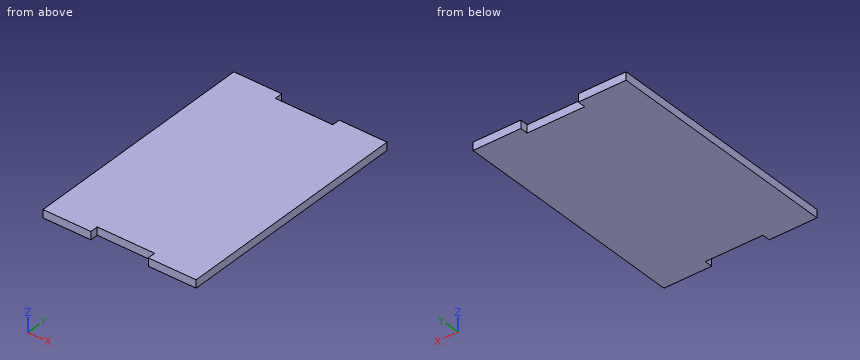
Autodesk Inventor part; units mm, degrees
ref_plane "YZ Plane" through (0, 0, 0) normal (1, 0, 0) x (0, 1, 0)
ref_plane "XZ Plane" through (0, 0, 0) normal (0, 1, 0) x (-1, 0, 0)
ref_plane "XY Plane" through (0, 0, 0) normal (0, 0, 1) x (1, 0, 0)
sketch "Sketch1" plane through (0, 0, 0) normal (0, 0, 1) x (1, 0, 0)
  line L0 (0, 2.8582) -> (0, -2.8582) construction
  line L1 (-5.7775, 0) -> (5.7775, 0) construction
  line L2 (0, 0) -> (96, 0)
  line L3 (96, 0) -> (96, -150)
  line L4 (96, -150) -> (0, -150)
  line L5 (0, -150) -> (0, 0)
  line L6 (0, 0) -> (30, 0)
  line L7 (30, 0) -> (66, 0)
  line L8 (0, -150) -> (30, -150)
  line L9 (30, 0) -> (66, 0)
  line L10 (66, 0) -> (66, -5)
  line L11 (66, -5) -> (30, -5)
  line L12 (30, -5) -> (30, 0)
  line L13 (30, -150) -> (66, -150)
  line L14 (66, -150) -> (66, -145)
  line L15 (66, -145) -> (30, -145)
  line L16 (30, -145) -> (30, -150)
  point P0 (66, 0)
  dimension "d1" = 96
  dimension "d2" = 150
  dimension "d3" = 30
  dimension "d5" = 30
  dimension "d7" = 36
  dimension "d8" = 5
  dimension "d9" = 36
  dimension "d10" = 5
  dimension "d13" = 30
extrude "Extrusion1" add sketch "Sketch1" along normal blind 5 contours L2 L12 L11 L10 L3 L4 L14 L15 L16 L5
properties part number "schuine plaat" material "S235"
Read the model definition and answer for the solid it produces. Units are mm, in the model's axes. Coordinates: 2 decimals unless noted, no trailing zeros. Write each loop counter-clockwise with the first axis right and the second up, starting at its lowest first coordinate (ties: lowest second). Pieces come first, ordered by that corner, then holes. Notation, with made-up numbers: (55.5, -29) -> (98.5, -29) arc R25 cw to (98.5, 2) -> close; hole circle Ø1 at (13.25, 49). An arc over 180 degrees is marked (long way). Write item = value, one per line.
(1) Section B-B on x = 46 is taken. Write down the section's boundary in (y, z), plus the area to 3 significant figures.
From the geometry:
outline = (-145, 0) -> (-5, 0) -> (-5, 5) -> (-145, 5) -> close
area = 700 mm2
(2) A straight line is drawn through the part: L1, parallel to Y at x = 47.5, z = 1.45. Find the intervals that lie inside material, in ascending order. Write a range as from..to.
From the geometry:
L1 = -145..-5
(3) Section A-A on z = 1.65 is taken. Write down the section's boundary in (x, y), plus the area to 3 significant figures.
From the geometry:
outline = (0, -150) -> (30, -150) -> (30, -145) -> (66, -145) -> (66, -150) -> (96, -150) -> (96, 0) -> (66, 0) -> (66, -5) -> (30, -5) -> (30, 0) -> (0, 0) -> close
area = 14,000 mm2
(4) Given pin 1 Ø1.5 at (x, z) = (47.5, 3) entering from -Y, flat-ended and moving along its own axis, determine where the tip first touches the part or whether it passes through.
From the geometry:
pin_1 = -145
